Here's how the part is built. I have some questions about the finished solid (model axes, mm). Face numbers are marked on the shaded views. A direction names the side the tool comes from. Coordinates: 2 decimals unless noted, no trailing zeros. Loops run counter-clockwise (first coordinate to the right, second up) from the corner with the lowest first, then second, coordinate; pieces in that order, holes last. Notation, with made-up numbers: (68, 28.5) -> (95, 28.5) arc R10 cw to (95, 37.5) -> close; hole circle Ø4 at (88.25, 4). An arc over 180 degrees is marked (long way). Answer as a JSON object with one key per item and string values. Group by question number.
1) I want a section at A-A (z = -19.5). Write out the boundary of the cut face in (x, y), then the cut area to 3 significant figures.
2) I want a section at C-C (z = 19). Write out the boundary of the cut face in (x, y), then the cut area to 3 significant figures.
3) If we mould it in two halves opening along X, with no side actions, what happens to the marked faces 5, 6 and 7? For each: +X half, -X half, draft (parallel to the pull), parting line (faces both ways), or undercut.
4) I want a section at D-D (x = 17). Write out the boundary of the cut face in (y, z), then the cut area to 3 significant figures.
5) I'm going to push flat-ended pins straight in: pin 1 (1.8 mm diameter, centred on x = 2.5, z = 33.3, fed in from -Y); pin 2 (3.5 mm diameter, centred on x = 42, z = 33.5, fed in from -Y); pin 3 (11 mm diameter, centred on y = -18, z = 39.5, fed in from -X); pin 4 (1 mm diameter, centred on x = 34, z = -6, fed in from -Y). Where does each tip first touch, or does it pass through?
6) Which directions (+Z, -Z, +X, -X, +Y, -Y) give clear straight access to the entire face, cutting with the end or side of a thin tool? Please do the marked faces 1, 2, 3 and 4.
7) I want a section at B-B (y = -20.25). Write out the boundary of the cut face in (x, z).
8) I need wall thicknesses on probe 1 along X at (y, z) = (-20.5, 33.3); probe 2 along X at (y, z) = (-2.85, -19.5); probe 3 along Z at (x, y) = (-3, -17). Which ranges of each line are inside material? Lowest first, please. Write a range as [from, to].
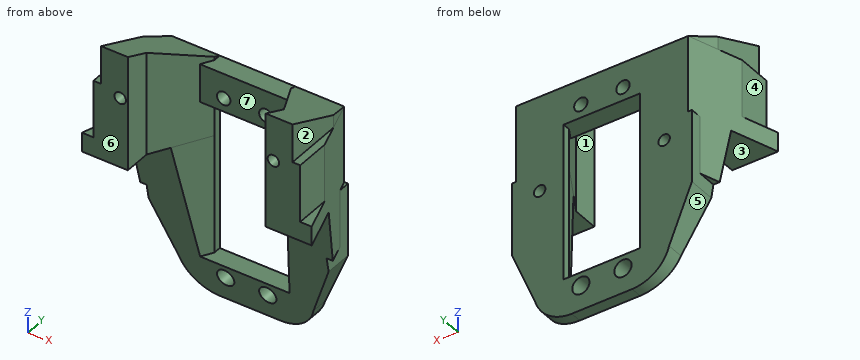
```python
from build123d import *

# Parameters (mm, degrees)
SALIENTE_EXTRUIR1_DEPTH = 35
CROQUIS6_R              = 2.25
CROQUIS6_W              = 20
CROQUIS6_H              = 25
CORTAR_EXTRUIR3_DEPTH   = 10
CROQUIS7_R              = 2.25
SALIENTE_EXTRUIR4_DEPTH = 15
CROQUIS8_R              = 1.5
CORTAR_EXTRUIR4_DEPTH   = 10
CORTAR_EXTRUIR8_DEPTH   = 50
CORTAR_EXTRUIR11_REACH  = 69.158
CORTAR_EXTRUIR12_DEPTH  = 16
CROQUIS13_W             = 6.081292266
CROQUIS13_H             = 9.753773429
CORTAR_EXTRUIR13_DEPTH  = 15
CORTAR_EXTRUIR14_DEPTH  = 63.5
CORTAR_EXTRUIR15_DEPTH  = 100
SALIENTE_EXTRUIR5_REACH = 69.158
CROQUIS16_W             = 15
CROQUIS16_H             = 10
CORTAR_EXTRUIR16_DEPTH  = 200
CORTAR_EXTRUIR17_DEPTH  = 200
SALIENTE_EXTRUIR7_DEPTH = 23.5
CROQUIS22_R             = 2.25
CORTAR_EXTRUIR19_DEPTH  = 47
CORTAR_EXTRUIR20_DEPTH  = 31
CROQUIS24_W             = 29.420485752
CROQUIS24_H             = 5
SALIENTE_EXTRUIR9_DEPTH = 10
CROQUIS25_R             = 1.75
CROQUIS25_R_2           = 1.5
CORTAR_EXTRUIR21_DEPTH  = 5


with BuildPart() as part:
    # Croquis1 → Saliente-Extruir1 (new body)
    with BuildSketch(Plane.XY):
        Polygon((0, 0), (45, 0), (52.5, -23), (40.5, -23), (40.5, -16.192411456), (32.5, -2), (12.5, -2), (4.5, -16), (4.5, -23), (-7.5, -23), align=None)
    extrude(amount=SALIENTE_EXTRUIR1_DEPTH)

    # Croquis6 → Cortar-Extruir3 (cut)
    with BuildSketch(Plane(origin=(0, 0, 0), x_dir=(1, 0, 0), z_dir=(0, 1, 0))):
        with Locations(Location((17, -28.5, 0), (0, 0, 180))):
            Circle(CROQUIS6_R)
        with Locations(Location((28, -28.5, 0), (0, 0, 270))):
            Circle(CROQUIS6_R)
        with Locations((22.5, -12.5)):
            Rectangle(CROQUIS6_W, CROQUIS6_H)
    extrude(amount=-CORTAR_EXTRUIR3_DEPTH, mode=Mode.SUBTRACT)

    # Croquis8 → Cortar-Extruir4 (cut)
    with BuildSketch(Plane(origin=(0, -23, 0), x_dir=(-1, 0, 0), z_dir=(0, -1, 0))):
        with Locations(Location((-2.5, -33.3, 0), (0, 0, 90))):
            Circle(CROQUIS8_R)
        with Locations(Location((-42.5, -33.3, 0), (0, 0, 270))):
            Circle(CROQUIS8_R)
    extrude(amount=-CORTAR_EXTRUIR4_DEPTH, mode=Mode.SUBTRACT)

    # Cortar-Extruir11: up to this plane
    cortar_extruir11_end = Plane(origin=(50, -15, 0), z_dir=(0, -0.9079593845004518, -0.41905817746174695))
    # Croquis11 → Cortar-Extruir11 (cut, up to the surface)
    with BuildSketch(Plane.XZ.offset(23), mode=Mode.PRIVATE) as cortar_extruir11_sk1:
        with BuildLine():
            Line((-7.5, 15), (-7.5, -3.030649644))
            Line((-7.5, -3.030649644), (52.5, -3.030649644))
            Line((52.5, -3.030649644), (52.5, 15))
            ThreePointArc((52.5, 15), (22.5, 5.553378231), (-7.5, 15))
        make_face()
    cortar_extruir11_tool1 = split(extrude(cortar_extruir11_sk1.sketch, amount=-CORTAR_EXTRUIR11_REACH, mode=Mode.PRIVATE), bisect_by=cortar_extruir11_end, keep=Keep.BOTH, mode=Mode.PRIVATE)
    add(cortar_extruir11_tool1.solids().sort_by_distance((22.5, -23, 3.105508))[0], mode=Mode.SUBTRACT)

    # Croquis13 → Cortar-Extruir13 (cut)
    with BuildSketch(Plane.XY.offset(35)):
        with Locations((-7.540646133, -18.123113286)):
            Rectangle(CROQUIS13_W, CROQUIS13_H)
        with Locations((52.540646133, -18.123113286)):
            Rectangle(CROQUIS13_W, CROQUIS13_H)
    extrude(amount=-CORTAR_EXTRUIR13_DEPTH, mode=Mode.SUBTRACT)

    # Croquis14 → Cortar-Extruir14 (cut, symmetric)
    with BuildSketch(Plane(origin=(0, 0, 0), x_dir=(0, 0, -1), z_dir=(1, 0, 0))):
        Polygon((-15, -11), (-15, -28.858785619), (26, -23), (26, -3), align=None)
    extrude(amount=CORTAR_EXTRUIR14_DEPTH, both=True, mode=Mode.SUBTRACT)

    # Saliente-Extruir5: up to this face of the body (flat: up to its plane)
    saliente_extruir5_end = Plane(part.part.faces().sort_by_distance((6.25, 0, 0.570087713))[0])
    # Croquis16 → Saliente-Extruir5 (add, up to the picked face)
    with BuildSketch(Plane.XZ.offset(23), mode=Mode.PRIVATE) as saliente_extruir5_sk1:
        with Locations((5, 40)):
            Rectangle(CROQUIS16_W, CROQUIS16_H)
    saliente_extruir5_tool1 = split(extrude(saliente_extruir5_sk1.sketch, amount=-SALIENTE_EXTRUIR5_REACH, mode=Mode.PRIVATE), bisect_by=saliente_extruir5_end, keep=Keep.BOTH, mode=Mode.PRIVATE)
    # Croquis16 → Saliente-Extruir5 (add, up to the picked face)
    with BuildSketch(Plane.XZ.offset(23), mode=Mode.PRIVATE) as saliente_extruir5_sk2:
        with Locations((40, 40)):
            Rectangle(CROQUIS16_W, CROQUIS16_H)
    saliente_extruir5_tool2 = split(extrude(saliente_extruir5_sk2.sketch, amount=-SALIENTE_EXTRUIR5_REACH, mode=Mode.PRIVATE), bisect_by=saliente_extruir5_end, keep=Keep.BOTH, mode=Mode.PRIVATE)
    add(saliente_extruir5_tool1.solids().sort_by(Axis((5, -23, 40), (0, 1, 0)))[0])
    add(saliente_extruir5_tool2.solids().sort_by(Axis((40, -23, 40), (0, 1, 0)))[0])

    # Croquis17 → Cortar-Extruir16 (cut)
    with BuildSketch(Plane.ZY.offset(2.5)):
        Polygon((35, 0), (45, -23), (45, 0), align=None)
    extrude(amount=-CORTAR_EXTRUIR16_DEPTH, mode=Mode.SUBTRACT)

    # Croquis18 → Cortar-Extruir17 (cut)
    with BuildSketch(Plane(origin=(0, 0, 35), x_dir=(-1, 0, 0), z_dir=(0, 0, -1))):
        Polygon((-32.5, -2), (-40.5, -16.192411456), (-40.5, -23), (-32.5, -23), align=None)
        Polygon((-12.5, -23), (-4.5, -23), (-4.5, -16), (-12.5, -2), align=None)
        Polygon((-47.5, -7.666666667), (-45, 0), (-47.5, 0), align=None)
        Polygon((2.5, 0), (0, 0), (2.5, -7.666666667), align=None)
    extrude(amount=-CORTAR_EXTRUIR17_DEPTH, mode=Mode.SUBTRACT)



with BuildPart() as body_2:
    # Croquis7 → Saliente-Extruir4 (new body)
    with BuildSketch(Plane(origin=(0, 0, 0), x_dir=(1, 0, 0), z_dir=(0, 1, 0))):
        with BuildLine():
            Line((12.5, 16), (32.5, 16))
            Line((32.5, 16), (32.5, 0))
            Line((32.5, 0), (45, 0))
            Line((45, 0), (40.044296858, 18.577458823))
            ThreePointArc((40.044296858, 18.577458823), (36.474189304, 23.930150952), (30.382169451, 26))
            Line((30.382169451, 26), (14.617830549, 26))
            ThreePointArc((14.617830549, 26), (8.525810696, 23.930150952), (4.955703142, 18.577458823))
            Line((4.955703142, 18.577458823), (0, 0))
            Line((0, 0), (12.5, 0))
            Line((12.5, 0), (12.5, 16))
        make_face()
        with Locations((28, 19.5)):
            Circle(CROQUIS7_R, mode=Mode.SUBTRACT)
        with Locations((17, 19.5)):
            Circle(CROQUIS7_R, mode=Mode.SUBTRACT)
    extrude(amount=-SALIENTE_EXTRUIR4_DEPTH)

    # Croquis10 → Cortar-Extruir8 (cut)
    with BuildSketch(Plane(origin=(0, 0, 0), x_dir=(0, 0, -1), z_dir=(1, 0, 0))):
        Polygon((0, -15), (26, -3), (26, 0), (28.244981963, 0), (28.244981963, -21.856093693), align=None)
    extrude(amount=CORTAR_EXTRUIR8_DEPTH, mode=Mode.SUBTRACT)

    # Croquis12 → Cortar-Extruir12 (cut)
    with BuildSketch(Plane.XY):
        Polygon((12.5, -2), (12.5, -7.5), (12.5, -22.325980529), (0.885153984, -22.325980529), align=None)
        Polygon((44.114846016, -22.325980529), (32.5, -22.325980529), (32.5, -7.5), (32.5, -2), align=None)
    extrude(amount=-CORTAR_EXTRUIR12_DEPTH, mode=Mode.SUBTRACT)

    # Croquis15 → Cortar-Extruir15 (cut, symmetric)
    with BuildSketch(Plane(origin=(0, 0, 0), x_dir=(0, 0, -1), z_dir=(1, 0, 0))):
        Polygon((-15, -23), (-15, -11), (26, -3), align=None)
    extrude(amount=CORTAR_EXTRUIR15_DEPTH, both=True, mode=Mode.SUBTRACT)


with BuildPart() as part_1:
    add(part.part)

    add(body_2.part)  # Saliente-Extruir7 merges body 2
    # Croquis20 → Saliente-Extruir7 (add, symmetric)
    with BuildSketch(Plane(origin=(22.5, 0, 0), x_dir=(0, 0, -1), z_dir=(1, 0, 0))):
        Polygon((-15, -11), (-15, 0), (26, 0), (26, -3), align=None)
    extrude(amount=SALIENTE_EXTRUIR7_DEPTH, both=True)

    # Croquis22 → Cortar-Extruir19 (cut)
    with BuildSketch(Plane(origin=(0, 0, 0), x_dir=(1, 0, 0), z_dir=(0, 1, 0))):
        with Locations(Location((17, 19.5, 0), (0, 0, 180))):
            Circle(CROQUIS22_R)
        with Locations(Location((28, 19.5, 0), (0, 0, 180))):
            Circle(CROQUIS22_R)
        Polygon((12.5, 0), (12.5, -25), (32.5, -25), (32.5, 0), (32.5, 16), (12.5, 16), align=None)
        with BuildLine():
            Line((4.955703142, 18.577458823), (-2.632555673, 0))
            Line((-2.632555673, 0), (-11.688532454, 0))
            Line((-11.688532454, 0), (-11.688532454, 31.257495622))
            Line((-11.688532454, 31.257495622), (0, 31.257495622))
            Line((0, 31.257495622), (45, 31.257495622))
            Line((45, 31.257495622), (54.896993635, 31.257495622))
            Line((54.896993635, 31.257495622), (58.873924375, 0))
            Line((58.873924375, 0), (47.632555673, 0))
            Line((47.632555673, 0), (40.044296858, 18.577458823))
            ThreePointArc((40.044296858, 18.577458823), (36.474189304, 23.930150952), (30.382169451, 26))
            Line((30.382169451, 26), (14.617830549, 26))
            ThreePointArc((14.617830549, 26), (8.525810696, 23.930150952), (4.955703142, 18.577458823))
        make_face()
    extrude(amount=-CORTAR_EXTRUIR19_DEPTH, mode=Mode.SUBTRACT)

    # Croquis23 → Cortar-Extruir20 (cut)
    with BuildSketch(Plane.XY.offset(15)):
        Polygon((7.357142857, -11), (12.5, -11), (12.5, -2), align=None)
        Polygon((37.573133641, -11), (32.5, -2), (32.5, -11), align=None)
    extrude(amount=-CORTAR_EXTRUIR20_DEPTH, mode=Mode.SUBTRACT)

    # Croquis24 → Saliente-Extruir9 (add)
    with BuildSketch(Plane.XY.offset(35)):
        with Locations((22.884581513, -2.5)):
            Rectangle(CROQUIS24_W, CROQUIS24_H)
    extrude(amount=-SALIENTE_EXTRUIR9_DEPTH)

    # Croquis25 → Cortar-Extruir21 (cut)
    with BuildSketch(Plane(origin=(0, 0, 0), x_dir=(1, 0, 0), z_dir=(0, 1, 0))):
        with Locations(Location((17, -28.5, 0), (0, 0, 180))):
            Circle(CROQUIS25_R)
        with Locations((28, -28.5)):
            Circle(CROQUIS25_R)
        with Locations(Location((6.253029256, -10.000000184, 0), (0, 0, 180))):
            Circle(CROQUIS25_R_2)
        with Locations((38.746970744, -10.000000184)):
            Circle(CROQUIS25_R_2)
    extrude(amount=-CORTAR_EXTRUIR21_DEPTH, mode=Mode.SUBTRACT)


solid = part_1.part
```
Determined:
{
 "1": {"outline": "(5.25, -4.27) -> (14.75, -4.27) -> (14.75, 0) -> (5.25, 0) -> close; (19.25, -4.27) -> (25.75, -4.27) -> (25.75, 0) -> (19.25, 0) -> close; (30.25, -4.27) -> (39.75, -4.27) -> (39.75, 0) -> (30.25, 0) -> close", "area": "109 mm^2"},
 "2": {"outline": "(-7.5, -23) -> (4.5, -23) -> (4.5, -16) -> (12.5, -2) -> (12.5, 0) -> (0, 0) -> close; (32.5, -2) -> (40.5, -16.19) -> (40.5, -23) -> (52.5, -23) -> (45, 0) -> (32.5, 0) -> close", "area": "524 mm^2"},
 "3": {"face 5": "-X half", "face 6": "draft", "face 7": "undercut"},
 "4": {"outline": "(-5, 25) -> (0, 25) -> (0, 26.75) -> (-5, 26.75) -> close; (-5, 30.25) -> (0, 30.25) -> (0, 35) -> (-5, 35) -> close; (-4.95, -16) -> (-4.71, -17.25) -> (0, -17.25) -> (0, -16) -> close; (-3.83, -21.75) -> (-3, -26) -> (0, -26) -> (0, -21.75) -> close", "area": "53.0 mm^2"},
 "5": {"pin 1": "y = -13", "pin 2": "y = -23", "pin 3": "x = -4.5", "pin 4": "y = -5.55"},
 "6": {"face 1": "+Z, -Z, -Y", "face 2": "+Z, +X, +Y, -Y", "face 3": "-Z, +X, -X, -Y", "face 4": "+Z, -X, +Y, -Y"},
 "7": {"outline": "(-6.6, 15) -> (4.5, 15) -> (4.5, 43.8) -> (-2.5, 43.8) -> (-2.5, 35) -> (-4.5, 35) -> (-4.5, 20) -> (-6.6, 20) -> close; (40.5, 15) -> (51.6, 15) -> (51.6, 20) -> (49.5, 20) -> (49.5, 35) -> (47.5, 35) -> (47.5, 43.8) -> (40.5, 43.8) -> close; hole circle Ø3 at (2.5, 33.3); hole circle Ø3 at (42.5, 33.3)"},
 "8": {"probe 1": "[-4.5, 1], [4, 4.5], [40.5, 41], [44, 49.5]", "probe 2": "[5.25, 14.75], [19.25, 25.75], [30.25, 39.75]", "probe 3": "[15, 35]"}
}
